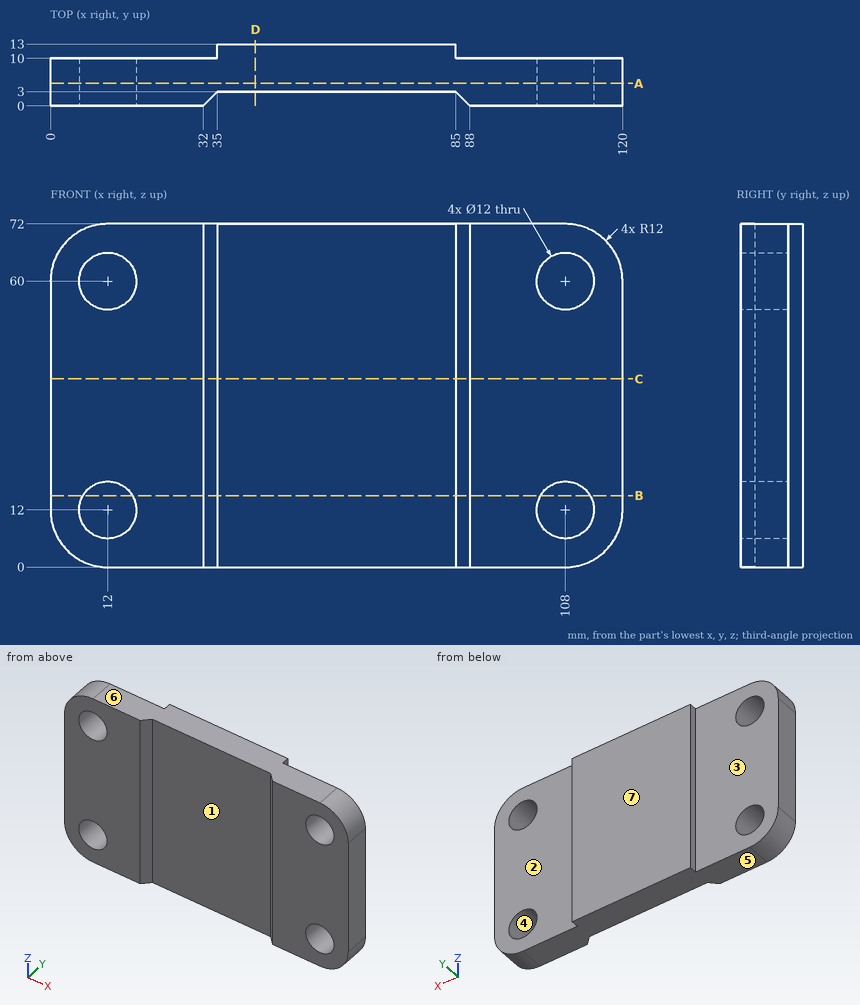
Input: dimensioned drawing with shaded views. Units: mm. Origin: part minimum x, y, z. A direction names the side the tool comes from. Round coordinates to 2 decimals unless told otherwise and drop trailing zeros. Order: outer loops, then holes, each group sorted by start corner. A loop starts at its lowest first (then second) coordinate and runs counter-clockwise, first axis right, second up. Notation, with made-up numbers: (-7, 82) -> (11, 82) arc R19 cw to (11, 119) -> close; hole circle Ø6 at (-6, 55.5). An arc over 180 degrees is marked (long way). One line per item, written item: value. Start each with the question number.
Q1. Access query for the marked faces 1, 2 and 3. Directions: +Z, -Z, +X, -X, +Y, -Y. A direction counts if a zero-diameter tool reaches every point of the face in a straight line with its end or side. Return the directions, or none.
Q2. Section query B-B (z = 15). Return the cut outline in (x, y).
Q3. Section query A-A (y = 4.75). Return the cut outline in (x, z).
Q4. Pin query (flat end, axial travel): pin 1 (2 mm diameter, centred on x = 26, z = 25, fed in from +Y); pin 2 (0.9 mm diameter, centred on y = 11.5, z = 53.5, fed in from +X); pin 3 (0.9 mm diameter, centred on y = 11, z = 52, fed in from -X). Return the tip coordinate at first contact, or that it passes through.
Q5. Section query D-D (x = 43). Return the cut outline in (y, z).
Q6. Material intervals for probe 1 along X at (y, z) = (7.5, 65); probe 2 along Y at (x, z) = (74.5, 37.5); probe 3 along Y at (x, z) = (108, 50), sorted ascending.
Q7. Draft query along Z for the marked faces 4, 5, 6 and 7. Return one class per face: pulls with the +Z half, pulls with the -Z half, needs draft (parallel to the pull), parting line crosses it, or undercut.
Q8. Section query C-C (z = 39.5). Return the cut outline in (x, y).
Findings below:
1. face 1: +Z, -Z, -Y
1. face 2: +Z, -Z, +X, +Y
1. face 3: +Z, -Z, -X, +Y
2. outline: (0, 0) -> (6.8, 0) -> (6.8, 10) -> (0, 10) -> close; (17.2, 0) -> (32, 0) -> (35, 3) -> (85, 3) -> (88, 0) -> (102.8, 0) -> (102.8, 10) -> (85, 10) -> (85, 13) -> (35, 13) -> (35, 10) -> (17.2, 10) -> close; (113.2, 0) -> (120, 0) -> (120, 10) -> (113.2, 10) -> close
3. outline: (0, 12) arc R12 ccw to (12, 0) -> (108, 0) arc R12 ccw to (120, 12) -> (120, 60) arc R12 ccw to (108, 72) -> (12, 72) arc R12 ccw to (0, 60) -> close; hole circle Ø12 at (12, 12); hole circle Ø12 at (12, 60); hole circle Ø12 at (108, 12); hole circle Ø12 at (108, 60)
4. pin 1: y = 10
4. pin 2: x = 85
4. pin 3: x = 35
5. outline: (3, 0) -> (13, 0) -> (13, 72) -> (3, 72) -> close
6. probe 1: 1.09 to 8.68, 15.32 to 104.68, 111.32 to 118.91
6. probe 2: 3 to 13
6. probe 3: 0 to 10
7. face 4: undercut
7. face 5: pulls with the -Z half
7. face 6: pulls with the +Z half
7. face 7: needs draft
8. outline: (0, 0) -> (32, 0) -> (35, 3) -> (85, 3) -> (88, 0) -> (120, 0) -> (120, 10) -> (85, 10) -> (85, 13) -> (35, 13) -> (35, 10) -> (0, 10) -> close
